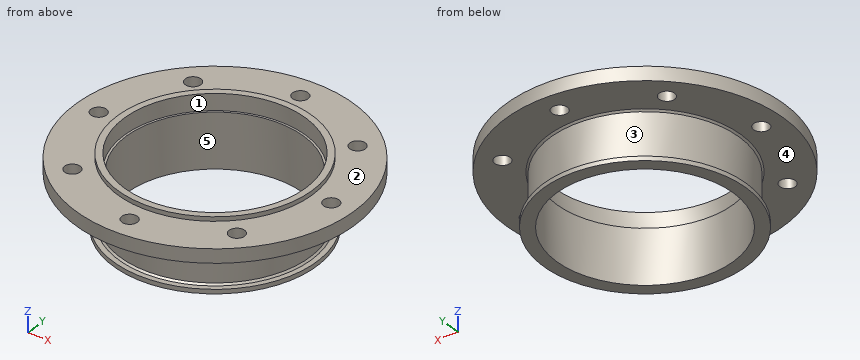
from build123d import *

# Parameters (mm, degrees)
SKETCH1_R           = 161
SKETCH1_R_2         = 102.5
BOSS_EXTRUDE1_DEPTH = 82
SKETCH2_R           = 9
CUT_EXTRUDE1_DEPTH  = 243.004132196
CIRPATTERN1_COUNT   = 8
SKETCH3_R           = 161
SKETCH3_R_2         = 109.5
CUT_EXTRUDE2_DEPTH  = 61
SKETCH4_R           = 117.5
SKETCH4_R_2         = 109.5
BOSS_EXTRUDE3_DEPTH = 5
CUT_EXTRUDE3_START  = -5
SKETCH6_R           = 161
SKETCH6_R_2         = 112.5
CUT_EXTRUDE3_DEPTH  = 5
CHAMFER1_SIZE       = 2
CHAMFER2_SIZE       = 2
SKETCH8_R           = 105
CUT_EXTRUDE5_DEPTH  = 19


with BuildPart() as part:
    # Sketch1 → Boss-Extrude1 (new body)
    with BuildSketch(Plane.XY):
        Circle(SKETCH1_R)
        Circle(SKETCH1_R_2, mode=Mode.SUBTRACT)
    extrude(amount=BOSS_EXTRUDE1_DEPTH)

    # Sketch2 → Cut-Extrude1 (cut, through all)
    with BuildSketch(Plane.XY.offset(82)):
        with Locations((0, 135)):
            Circle(SKETCH2_R)
    cut_extrude1 = extrude(amount=-CUT_EXTRUDE1_DEPTH, mode=Mode.SUBTRACT)

    # CirPattern1: Cut-Extrude1 ×8 about axis
    cirpattern1_axis = Axis((0, 0, 0), (0, 0, 1))
    for i in range(1, CIRPATTERN1_COUNT):
        add(cut_extrude1.rotate(cirpattern1_axis, i * 360 / CIRPATTERN1_COUNT), mode=Mode.SUBTRACT)

    # Sketch3 → Cut-Extrude2 (cut)
    with BuildSketch(Plane(origin=(0, 0, 0), x_dir=(-1, 0, 0), z_dir=(0, 0, -1))):
        Circle(SKETCH3_R)
        Circle(SKETCH3_R_2, mode=Mode.SUBTRACT)
    extrude(amount=-CUT_EXTRUDE2_DEPTH, mode=Mode.SUBTRACT)

    # Sketch4 → Boss-Extrude3 (add)
    with BuildSketch(Plane(origin=(0, 0, 0), x_dir=(-1, 0, 0), z_dir=(0, 0, -1))):
        Circle(SKETCH4_R)
        Circle(SKETCH4_R_2, mode=Mode.SUBTRACT)
    extrude(amount=-BOSS_EXTRUDE3_DEPTH)

    # Sketch6 → Cut-Extrude3 (cut)
    with BuildSketch(Plane.XY.offset(82).offset(CUT_EXTRUDE3_START)):
        with Locations(Location((0, 0, 0), (0, 0, 180))):
            Circle(SKETCH6_R)
        Circle(SKETCH6_R_2, mode=Mode.SUBTRACT)
    extrude(amount=CUT_EXTRUDE3_DEPTH, mode=Mode.SUBTRACT)

    # Chamfer1
    chamfer1_edges = [part.edges().sort_by_distance(p)[0] for p in [
        (109.5, 0, 5),
    ]]
    chamfer(chamfer1_edges, length=CHAMFER1_SIZE)

    # Chamfer2
    chamfer2_edges = [part.edges().sort_by_distance(p)[0] for p in [
        (109.5, 0, 61),
    ]]
    chamfer(chamfer2_edges, length=CHAMFER2_SIZE)

    # Sketch8 → Cut-Extrude5 (cut)
    with BuildSketch(Plane.XY.offset(82)):
        Circle(SKETCH8_R)
    extrude(amount=-CUT_EXTRUDE5_DEPTH, mode=Mode.SUBTRACT)


solid = part.part
Verification items for the finished model (mm, model axes). Face numbers are marked on the shaded views. A direction names the side the tool comes from. Coordinates: 2 decimals unless noted, no trailing zeros. Write each loop counter-clockwise with the first axis right and the second up, starting at its lowest first coordinate (ties: lowest second). Pieces come first, ordered by that corner, then holes. Notation, with made-up numbers: (53.5, 45.5) -> (83.5, 45.5) arc R16 cw to (83.5, 50.5) -> close; hole circle Ø1 at (21.5, 10.25). An arc over 180 degrees is marked (long way). One line per item, written item: value. Start each with the question number.
Q1. Cross-section at C-C on z = 44. Enter the section's corners in (x, y).
Q2. Cross-section at A-A on x = 135. Enter the section's corners in (y, z).
Q3. Thickness scan on L1, parallel to Y at x = -0.5, z = 21; L2, parallel to Z at x = 119, y = -17.5; L3, parallel to Y at x = 69.5, z = 52. Record the ranges inside material, lowest first. Write a range as from..to.
Q4. Cross-section at D-D on x = 0. State how many separate pieces and enclosed holes the cut face has, and give its area (3 significant figures).
Q5. Access from +Z, -Z, +X, -X, +Y, -Y to the whole of each face (thin tool, end or side, straight path). Record for the marked faces 4 and 5.
Q6. Mould release check, pull along Z, two halves, no side actions. Record for the marked faces 1, 2 and 3: pulls with the +Z half, pulls with the -Z half, needs draft (parallel to the pull), parting line crosses it, or undercut.
Q7. Go/stop test with flat-tipped pins: P1, Ø2, axis at y = -18.5, z = 32, coming from the -X side; P2, Ø1.5, axis at y = 88, z = 41.5, coming from the -X side; P3, Ø1.5, axis at x = -31, y = 128.5, coming from the -Z side. Record where each tip stops, or that it passes through.
Checked values:
1. outline: circle Ø219 at (0, 0); hole circle Ø205 at (0, 0)
2. outline: (-87.73, 61) -> (-9, 61) -> (-9, 77) -> (-87.73, 77) -> close; (9, 61) -> (87.73, 61) -> (87.73, 77) -> (9, 77) -> close
3. L1: y = -109.5..-102.5, 102.5..109.5
3. L2: z = 61..77
3. L3: y = -84.62..-75.34, 75.34..84.62
4. separate pieces: 4
4. enclosed holes: 0
4. area: 2,240 mm²
5. face 4: none
5. face 5: +Z, -Z
6. face 1: needs draft
6. face 2: pulls with the +Z half
6. face 3: undercut
7. P1: stops at x = -108.09
7. P2: stops at x = -66.16
7. P3: stops at z = 61
